Print and shaded views of the part. All mm, measured from the part's lowest x, y and z. A direction names the side the tool comes from. Give positions to 0.01 mm unless a question says otherwise; leave off trailing zeros. Write each loop counter-clockwise with the first axis right and the second up, starting at its lowest first coordinate (ties: lowest second). Pieces come first, ordered by that corner, then holes. Notation, with made-up numbers: M 51.5,9.5 L 109.5,9.5 A17 ccw 109.5,33.5 Z; hole C 20,-6.5 d11. An arc over 180 degrees is marked long. One line per question, with ' | ' between items. Start each with the question number.
1. Wall check: L1, parallel to Y at x = 5.5, z = 1.25; L2, parallel to Y at x = 2.5, z = 24; L3, parallel to Z at x = 12.5, y = 2.75. Give the ranges that are in metal, low to high.
2. Flat gauge pins, fed straight in: pin 1 (9 mm diameter, centred on x = 24.5, z = 21, fed in from -Y); pin 2 (3.5 mm diameter, centred on x = 5.5, y = 4, fed in from +Z). Where does each tip first touch, or does it go through?
3. Cut at D-D, the plane z = 16. Write the cut outline in (x, y), then the cut area to 3 significant figures.
4. Cut at C-C, the plane x = 8.5. Write the cut outline in (y, z), then the cut area to 3 significant figures.
5. Which spindle directions (+Z, -Z, +X, -X, +Y, -Y) get a long thin tool onto all of the face, cutting with end or side? Do the marked faces 1 and 2. Say none if no direction does.
6. Cut at B-B, the plane x = 29.5. Write the cut outline in (y, z).
7. Cut at A-A, the plane y = 4. Write the cut outline in (x, z).
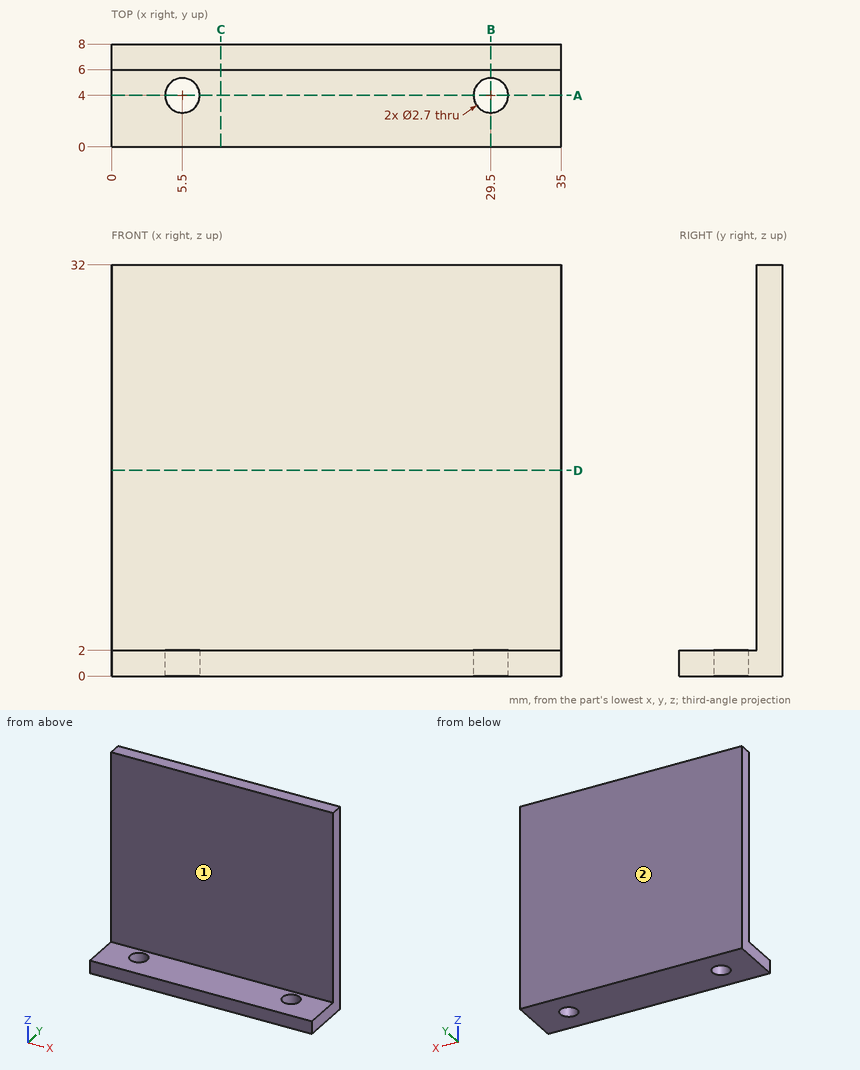
Here are the results:
1) L1: 0 to 2.65, 5.35 to 8 | L2: 6 to 8 | L3: 0 to 2
2) pin 1: y = 6 | pin 2: z = 2
3) outline: M 0,6 L 35,6 L 35,8 L 0,8 Z | area: 70.0 mm^2
4) outline: M 0,0 L 8,0 L 8,32 L 6,32 L 6,2 L 0,2 Z | area: 76.0 mm^2
5) face 1: +Z, +X, -X, -Y | face 2: +Z, -Z, +X, -X, +Y
6) outline: M 0,0 L 2.65,0 L 2.65,2 L 0,2 Z; M 5.35,0 L 8,0 L 8,32 L 6,32 L 6,2 L 5.35,2 Z
7) outline: M 0,0 L 4.15,0 L 4.15,2 L 0,2 Z; M 6.85,0 L 28.15,0 L 28.15,2 L 6.85,2 Z; M 30.85,0 L 35,0 L 35,2 L 30.85,2 Z
